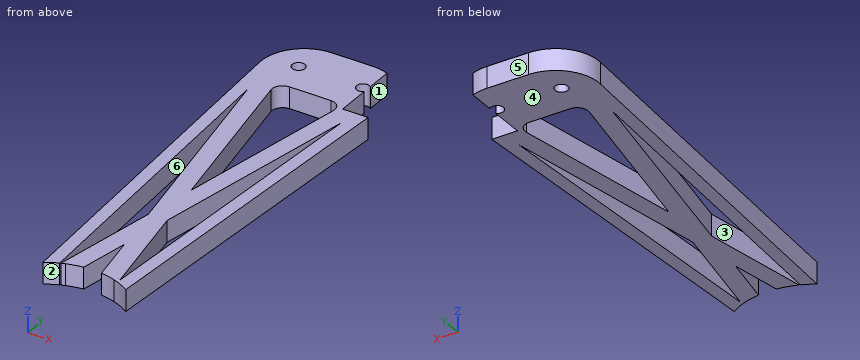
```python
from build123d import *

# Parameters (mm, degrees)
SKETCH1_R           = 3
BOSS_EXTRUDE2_DEPTH = 10
FILLET1_R           = 20
FILLET2_R           = 20
CUT_EXTRUDE1_START  = -10
CUT_EXTRUDE1_DEPTH  = 10
FILLET3_R           = 5
CUT_EXTRUDE3_START  = -10
SKETCH5_W           = 12
SKETCH5_H           = 10
CUT_EXTRUDE3_DEPTH  = 10


with BuildPart() as part:
    # Sketch1 → Boss-Extrude2 (new body)
    with BuildSketch(Plane.XY):
        with BuildLine():
            Line((-30, 15.770412854), (-30, 0))
            Line((-30, 0), (-17.5, -210))
            ThreePointArc((-17.5, -210), (0, -227.5), (17.5, -210))
            Line((17.5, -210), (30, 0))
            Line((30, 0), (30, 15.770412854))
            Line((30, 15.770412854), (-30, 15.770412854))
        make_face()
        with Locations((-15, 0)):
            Circle(SKETCH1_R, mode=Mode.SUBTRACT)
        with Locations((15, 0)):
            Circle(SKETCH1_R, mode=Mode.SUBTRACT)
        Polygon((0, -205), (6, -205), (6, -215), (-6, -215), (-6, -205), align=None, mode=Mode.SUBTRACT)
    extrude(amount=BOSS_EXTRUDE2_DEPTH)

    # Fillet1
    fillet1_edges = [part.edges().sort_by_distance(p)[0] for p in [
        (-30, 15.770412854, 5),
    ]]
    fillet(fillet1_edges, radius=FILLET1_R)

    # Fillet2
    fillet2_edges = [part.edges().sort_by_distance(p)[0] for p in [
        (30, 15.770412854, 5),
    ]]
    fillet(fillet2_edges, radius=FILLET2_R)

    # Sketch4 → Cut-Extrude1 (cut)
    with BuildSketch(Plane.XY.offset(10).offset(CUT_EXTRUDE1_START)):
        Polygon((-15.651797422, -15), (0.190220551, -102.160979768), (15.643622882, -15), (15, -15), align=None)
        Polygon((-22.473027071, -25.6531452), (-13.367328465, -178.628881795), (-4.134156204, -126.551525408), align=None)
        Polygon((22.230419841, -27.161313899), (4.615986353, -126.511039477), (13.430162671, -175.005634359), align=None)
        with BuildLine():
            Line((0.291609598, -150.901585116), (-7.372445375, -194.128735111))
            ThreePointArc((-7.372445375, -194.128735111), (0.476576628, -192.506490497), (8.225632191, -194.553674383))
            Line((8.225632191, -194.553674383), (0.291609598, -150.901585116))
        make_face()
    extrude(amount=CUT_EXTRUDE1_DEPTH, mode=Mode.SUBTRACT)

    # Fillet3
    fillet3_edges = [part.edges().sort_by_distance(p)[0] for p in [
        (8.225632191, -194.553674383, 5),
        (-7.372445375, -194.128735111, 5),
        (-15.651797422, -15, 5),
        (15.643622882, -15, 5),
    ]]
    fillet(fillet3_edges, radius=FILLET3_R)

    # Sketch5 → Cut-Extrude3 (cut)
    # profile 1 of 10: a face of its own
    with BuildSketch(Plane.XY.offset(10).offset(CUT_EXTRUDE3_START)):
        with BuildLine():
            Line((-4.167269409, -176.050756454), (-4.122092315, -175.795946561))
            Line((-4.122092315, -175.795946561), (-11.228656567, -175.795946561))
            ThreePointArc((-11.228656567, -175.795946561), (-12.106175916, -176.096600396), (-12.975657802, -176.419763184))
            Line((-12.975657802, -176.419763184), (-13.345719148, -178.506999951))
            ThreePointArc((-13.345719148, -178.506999951), (-8.842198544, -176.958619935), (-4.167269409, -176.050756454))
        make_face()
    # profile 2 of 10: a face of its own
    with BuildSketch(Plane.XY.offset(10).offset(CUT_EXTRUDE3_START)):
        with BuildLine():
            ThreePointArc((-13.486799408, -176.621769943), (-16.46588928, -177.986339006), (-19.308563513, -179.61613298))
            Line((-19.308563513, -179.61613298), (-19.185515511, -181.683339422))
            ThreePointArc((-19.185515511, -181.683339422), (-16.356398794, -179.96026814), (-13.373872309, -178.518945203))
            Line((-13.373872309, -178.518945203), (-13.486799408, -176.621769943))
        make_face()
    # profile 3 of 10: a face of its own
    with BuildSketch(Plane.XY.offset(10).offset(CUT_EXTRUDE3_START)):
        with BuildLine():
            Line((-4.122092315, -175.795946561), (-3.840092025, -174.205395752))
            ThreePointArc((-3.840092025, -174.205395752), (-7.576229867, -174.806240028), (-11.228656567, -175.795946561))
            Line((-11.228656567, -175.795946561), (-4.122092315, -175.795946561))
        make_face()
    # profile 4 of 10: a face of its own
    with BuildSketch(Plane.XY.offset(10).offset(CUT_EXTRUDE3_START)):
        with BuildLine():
            Line((4.816305425, -175.795946561), (11.228656567, -175.795946561))
            ThreePointArc((11.228656567, -175.795946561), (7.921392788, -174.882318751), (4.542172021, -174.287695771))
            Line((4.542172021, -174.287695771), (4.816305425, -175.795946561))
        make_face()
    # profile 5 of 10: a face of its own
    with BuildSketch(Plane.XY.offset(10).offset(CUT_EXTRUDE3_START)):
        with BuildLine():
            ThreePointArc((19.308563513, -179.61613298), (15.387621929, -177.454323), (11.228656567, -175.795946561))
            Line((11.228656567, -175.795946561), (4.816305425, -175.795946561))
            Line((4.816305425, -175.795946561), (4.879901452, -176.145844664))
            ThreePointArc((4.879901452, -176.145844664), (12.347146855, -178.102269105), (19.185515511, -181.683339422))
            Line((19.185515511, -181.683339422), (19.308563513, -179.61613298))
        make_face()
    # profile 6 of 10: a face of its own
    with BuildSketch(Plane.XY.offset(10).offset(CUT_EXTRUDE3_START)):
        with BuildLine():
            Line((18.887385797, -186.691918617), (19.185515511, -181.683339422))
            ThreePointArc((19.185515511, -181.683339422), (12.347146855, -178.102269105), (4.879901452, -176.145844664))
            Line((4.879901452, -176.145844664), (5.679005105, -180.54242201))
            ThreePointArc((5.679005105, -180.54242201), (12.662186526, -182.803142969), (18.887385797, -186.691918617))
        make_face()
    # profile 7 of 10: a face of its own
    with BuildSketch(Plane.XY.offset(10).offset(CUT_EXTRUDE3_START)):
        with BuildLine():
            Line((17.5, -210), (18.887385797, -186.691918617))
            ThreePointArc((18.887385797, -186.691918617), (12.662186526, -182.803142969), (5.679005105, -180.54242201))
            Line((5.679005105, -180.54242201), (6.795310384, -186.684206595))
            ThreePointArc((6.795310384, -186.684206595), (5.577551358, -190.939561161), (1.45903868, -192.560928748))
            ThreePointArc((1.45903868, -192.560928748), (0.292984986, -192.502452749), (-0.874372768, -192.521857299))
            ThreePointArc((-0.874372768, -192.521857299), (-4.874459747, -190.834989527), (-6.047413252, -186.655228912))
            Line((-6.047413252, -186.655228912), (-4.940068564, -180.409533248))
            ThreePointArc((-4.940068564, -180.409533248), (-12.320876057, -182.646828096), (-18.887385797, -186.691918617))
            Line((-18.887385797, -186.691918617), (-17.5, -210))
            ThreePointArc((-17.5, -210), (0, -227.5), (17.5, -210))
        make_face()
        with Locations((0, -210)):
            Rectangle(SKETCH5_W, SKETCH5_H, mode=Mode.SUBTRACT)
    # profile 8 of 10: a face of its own
    with BuildSketch(Plane.XY.offset(10).offset(CUT_EXTRUDE3_START)):
        with BuildLine():
            Line((-4.940068564, -180.409533248), (-4.167269409, -176.050756454))
            ThreePointArc((-4.167269409, -176.050756454), (-8.842198544, -176.958619935), (-13.345719148, -178.506999951))
            Line((-13.345719148, -178.506999951), (-13.367328465, -178.628881795))
            Line((-13.367328465, -178.628881795), (-13.373872309, -178.518945203))
            ThreePointArc((-13.373872309, -178.518945203), (-16.356398794, -179.96026814), (-19.185515511, -181.683339422))
            Line((-19.185515511, -181.683339422), (-18.887385797, -186.691918617))
            ThreePointArc((-18.887385797, -186.691918617), (-12.320876057, -182.646828096), (-4.940068564, -180.409533248))
        make_face()
    # profile 9 of 10: a face of its own
    with BuildSketch(Plane.XY.offset(10).offset(CUT_EXTRUDE3_START)):
        with BuildLine():
            ThreePointArc((17, 2.236067977), (17.738612788, 1.224744871), (18, 0))
            Line((18, 0), (29.260488635, 0))
            ThreePointArc((29.260488635, 0), (24.938968919, 8.738256866), (17, 14.39559177))
            Line((17, 14.39559177), (17, 2.236067977))
        make_face()
    # profile 10 of 10: a face of its own
    with BuildSketch(Plane.XY.offset(10).offset(CUT_EXTRUDE3_START)):
        with BuildLine():
            Line((29.260488635, 0), (18, 0))
            ThreePointArc((18, 0), (17.738612788, -1.224744871), (17, -2.236067977))
            Line((17, -2.236067977), (17, -18))
            Line((17, -18), (28.928571429, -18))
            Line((28.928571429, -18), (29.677502384, -5.417959945))
            ThreePointArc((29.677502384, -5.417959945), (29.653859351, -2.694751229), (29.260488635, 0))
        make_face()
    extrude(amount=CUT_EXTRUDE3_DEPTH, mode=Mode.SUBTRACT)


solid = part.part
```
Geometry: final body of the model. Coordinates: model frame, mm. Face numbers are marked on the shaded views. A direction names the side the tool comes from. Round coordinates to 2 decimals unless told otherwise and drop trailing zeros. Order: outer loops, then holes, each group sorted by start corner. A loop starts at its lowest first (then second) coordinate and runs counter-clockwise, first axis right, second up. Notation, with made-up numbers: M -1.5,52.25 L 56.5,52.25 A33 ccw 56.5,80.25 Z; hole C 37.5,53.25 d2. An arc over 180 degrees is marked long. Use one line per item in the form item = value. Start each with the question number.
Q1. Cut plane C-C (z = 2). Count the separate pieces of the cut face and the enclosed holes in it, and give its area (3 significant figures).
Q2. Material intervals for line 1 (X direction, y = -131.5, z = 1.5); line 2 (X direction, y = -108.5, z = 5.25); line 3 (X direction, y = -84, z = 3.5), sorted ascending. Write a range as [from, to].
Q3. Mould query, pull axis Y, two halves, no side actions, for the marked faces 4, 5 and 6. Classes: +Y half, -Y half, draft (parallel to the pull), parting line (faces both ways), or undercut.
Q4. Pin query (flat end, axial travel): pin 1 Ø1.5 at (y, z) = (-41, 8.5) entering from +X; pin 2 Ø3 at (y, z) = (-10.5, 7) entering from +X; pin 3 Ø1 at (x, z) = (-18.5, 2) entering from -Y; pin 4 Ø8 at (x, y) = (-15, 0) entering from +Z. Return the tip coordinate at first contact, or that it passes through.
Q5. Cut plane B-B (y = -55.5). Return loops of the section in (x, z).
Q6. Cut plane A-A (y = -110.5). Return loops of the section in (x, z).
Q7. Access query for the marked faces 1, 2 and 3. Directions: +Z, -Z, +X, -X, +Y, -Y. A direction counts if a zero-diameter tool reaches every point of the face in a straight line with its end or side. Return the directions, or none.
Geometry results:
q1.separate_pieces = 1
q1.enclosed_holes = 3
q1.area = 5,830 mm^2
q2.line_1 = [-22.17, -16.17], [-5.01, 5.52], [16.02, 22.17]
q2.line_2 = [-23.54, -17.54], [-7.42, 7.81], [17.39, 23.54]
q2.line_3 = [-25, -19], [-11.87, -3.11], [3.41, 12.15], [18.85, 25]
q3.face_4 = draft
q3.face_5 = +Y half
q3.face_6 = undercut
q4.pin_1 = 27.6
q4.pin_2 = 17
q4.pin_3 = -179.42
q4.pin_4 = 10
q5.outline = M -26.7,0 L -20.7,0 L -20.7,10 L -26.7,10 Z; M -17.05,0 L -8.29,0 L -8.29,10 L -17.05,10 Z; M 8.46,0 L 17.21,0 L 17.21,10 L 8.46,10 Z; M 20.54,0 L 26.7,0 L 26.7,10 L 20.54,10 Z
q6.outline = M -23.42,0 L -17.42,0 L -17.42,10 L -23.42,10 Z; M -7.05,0 L 7.45,0 L 7.45,10 L -7.05,10 Z; M 17.27,0 L 23.42,0 L 23.42,10 L 17.27,10 Z
q7.face_1 = +Z, -Z, +X, +Y
q7.face_2 = +Z, -Z, -Y
q7.face_3 = +Z, -Z
